Build history of the part. All positions in model axes, mm. Face numbers are marked on the shaded views. A direction names the side the tool comes from. Round coordinates to 2 decimals unless told otherwise and drop trailing zeros. Write each loop counter-clockwise with the first axis right and the second up, starting at its lowest first coordinate (ties: lowest second). Pieces come first, ordered by that corner, then holes.
Item 1: Band-saw the part on A-A, the plane x = 0. Write the cut outline in (y, z) (3 decimals).
Item 2: Band-saw the part on C-C, the plane y = 16. Write the cut outline in (x, z), then the cut area to 3 significant figures.
Item 3: 3-axis set-ups, long thin cutter, end or side, ignore diameter. For the marked faces 1, 2 and 3: which of +Z, -Z, +X, -X, +Y, -Y reach the whole face in a straight line?
Item 4: Mould opens along Z. For the marked faces 4, 5, 6 and 7 say: +Z half, -Z half, draft (parallel to the pull), parting line (faces both ways), or undercut.
Item 5: Band-saw the part on D-D, the plane y = 45. Write the cut outline in (x, z).
Item 6: Wall check: probe 1 along Z at (x, y) = (0, 3); probe 2 along X at (y, z) = (39, 0); probe 3 along Z at (x, y) = (0, 36). Give the ranges that are in metal, low to high.
Item 7: Drop flat-ended pins along their axis: pin 1 Ø13.5 at (x, z) = (-7.5, -4) entering from +Y; pin 2 Ø4 at (x, y) = (2, 38) entering from +Z; pin 3 Ø4 at (x, z) = (6.5, -31.5) entering from -Y; pin 4 Ø3 at (x, z) = (8, -36.5) entering from +Y. Give the stop position or say it passes through.
Item 8: Band-saw the part on B-B, the plane y = 34. Write the cut outline in (x, z), then the cut area to 3 significant figures.
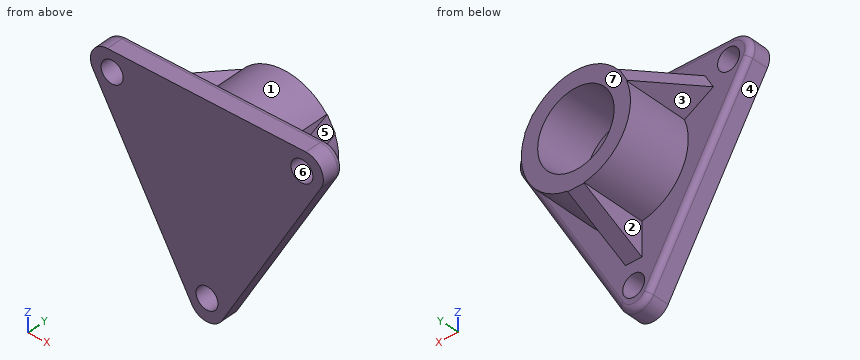
```python
from build123d import *

# Parameters (mm, degrees)
SKETCH1_R           = 6.369474113
SKETCH1_R_2         = 6.364401416
SKETCH1_R_3         = 6.413225573
BOSS_EXTRUDE2_DEPTH = 12.7
FILLET5_R           = 9.906
FILLET6_R           = 10.16
FILLET7_R           = 10.16
FILLET8_R           = 3.175
SKETCH2_R           = 31.696441514
BOSS_EXTRUDE3_DEPTH = 38.1
SKETCH3_R           = 22.193645705
CUT_EXTRUDE1_DEPTH  = 31.75
BOSS_EXTRUDE4_DEPTH = 4.7625
BOSS_EXTRUDE6_DEPTH = 9.525
CIRPATTERN1_COUNT   = 3


with BuildPart() as part:
    # Sketch1 → Boss-Extrude2 (new body)
    with BuildSketch(Plane(origin=(0, 0, 0), x_dir=(1, 0, 0), z_dir=(0, 1, 0))):
        Polygon((0, 86.591919686), (-74.990802211, -43.295959843), (74.990802211, -43.295959843), align=None)
        with Locations((0, 63.638807052)):
            Circle(SKETCH1_R, mode=Mode.SUBTRACT)
        with Locations((55.112823574, -31.819403526)):
            Circle(SKETCH1_R_2, mode=Mode.SUBTRACT)
        with Locations((-55.112823574, -31.819403526)):
            Circle(SKETCH1_R_3, mode=Mode.SUBTRACT)
    extrude(amount=BOSS_EXTRUDE2_DEPTH)

    # Fillet5
    fillet5_edges = [part.edges().sort_by_distance(p)[0] for p in [
        (-74.990802211, 6.35, 43.295959843),
    ]]
    fillet(fillet5_edges, radius=FILLET5_R)

    # Fillet6
    fillet6_edges = [part.edges().sort_by_distance(p)[0] for p in [
        (74.990802211, 6.35, 43.295959843),
    ]]
    fillet(fillet6_edges, radius=FILLET6_R)

    # Fillet7
    fillet7_edges = [part.edges().sort_by_distance(p)[0] for p in [
        (0, 6.35, -86.591919686),
    ]]
    fillet(fillet7_edges, radius=FILLET7_R)

    # Fillet8
    fillet8_edges = [part.edges().sort_by_distance(p)[0] for p in [
        (-0.219970453, 12.7, 43.295959843),
        (-66.411954561, 12.7, 38.342959843),
        (37.495401105, 12.7, -21.647979922),
        (66.191984109, 12.7, 38.215959843),
        (-37.605386332, 12.7, -21.457479922),
        (0, 12.7, -76.431919686),
    ]]
    fillet(fillet8_edges, radius=FILLET8_R)

    # Sketch2 → Boss-Extrude3 (add)
    with BuildSketch(Plane(origin=(0, 12.7, 0), x_dir=(1, 0, 0), z_dir=(0, 1, 0))):
        Circle(SKETCH2_R)
    extrude(amount=BOSS_EXTRUDE3_DEPTH)

    # Sketch3 → Cut-Extrude1 (cut)
    with BuildSketch(Plane(origin=(0, 50.8, 0), x_dir=(1, 0, 0), z_dir=(0, 1, 0))):
        Circle(SKETCH3_R)
    extrude(amount=-CUT_EXTRUDE1_DEPTH, mode=Mode.SUBTRACT)

    # Sketch6 → Boss-Extrude4 (add)
    with BuildSketch(Plane(origin=(0, 0, 0), x_dir=(-0.866025404, 0, 0.5), z_dir=(-0.5, 0, -0.866025404))):
        Polygon((31.696441514, 12.7), (50.655531139, 12.7), (31.696441514, 50.8), (28.066895326, 50.8), (28.066895326, 12.7), align=None)
    extrude(amount=BOSS_EXTRUDE4_DEPTH)

    # Sketch8 → Boss-Extrude6 (add)
    with BuildSketch(Plane(origin=(-2.38125, 0, -4.124445986), x_dir=(-0.866025404, 0, 0.5), z_dir=(-0.5, 0, -0.866025404))):
        Polygon((31.005254456, 12.578941577), (50.655531139, 12.7), (31.696441514, 50.8), (27.148658098, 50.8), (27.148658098, 12.578941577), align=None)
    boss_extrude6 = extrude(amount=-BOSS_EXTRUDE6_DEPTH)

    # CirPattern1: Boss-Extrude6 ×3 about axis
    cirpattern1_axis = Axis((0, 0, 0), (0, 1, 0))
    for i in range(1, CIRPATTERN1_COUNT):
        add(boss_extrude6.rotate(cirpattern1_axis, i * 360 / CIRPATTERN1_COUNT))


solid = part.part
```
Results:
1. outline: (0, -76.432) - (9.525, -76.432) arc R3.175 ccw to (12.7, -73.257) - (12.7, -70.008) - (0, -70.008) - close; (0, -57.269) - (12.7, -57.269) - (12.7, -50.656) - (50.8, -31.696) - (50.8, -22.194) - (19.05, -22.194) - (19.05, 22.194) - (50.8, 22.194) - (50.8, 31.696) - (12.7, 31.696) - (12.7, 40.121) arc R3.175 ccw to (9.525, 43.296) - (0, 43.296) - close
2. outline: (-44.83, 20.38) - (-29.52, 11.54) arc R31.7 ccw to (-4.76, -31.34) - (-4.76, -49.01) - (4.76, -49.01) - (4.76, -31.34) arc R31.7 ccw to (29.52, 11.54) - (44.83, 20.38) - (40.07, 28.63) - (24.76, 19.79) arc R31.7 ccw to (-24.76, 19.79) - (-40.07, 28.63) - close
2. area: 3,650 mm2
3. face 1: +Z, +Y
3. face 2: -Z, -X, +Y
3. face 3: -X, +Y
4. face 4: -Z half
4. face 5: +Z half
4. face 6: undercut
4. face 7: draft
5. outline: (-32.33, 13.17) - (-29.52, 11.54) arc R31.7 ccw to (-4.76, -31.34) - (-4.76, -34.58) - (4.76, -34.58) - (4.76, -31.34) arc R31.7 ccw to (29.52, 11.54) - (32.33, 13.17) - (27.57, 21.42) - (24.76, 19.79) arc R31.7 ccw to (-24.76, 19.79) - (-27.57, 21.42) - close; hole circle Ø44.39 at (0, 0)
6. probe 1: z = -76.43 to -70.01, -57.27 to 43.3
6. probe 2: x = -31.7 to -22.19, 22.19 to 31.7
6. probe 3: z = -39.06 to -22.19, 22.19 to 31.7
7. pin 1: stops at y = 19.05
7. pin 2: stops at z = 31.7
7. pin 3: stops at y = 0
7. pin 4: stops at y = 12.7
8. outline: (-37.07, 15.9) - (-29.52, 11.54) arc R31.7 ccw to (-4.76, -31.34) - (-4.76, -40.06) - (4.76, -40.06) - (4.76, -31.34) arc R31.7 ccw to (29.52, 11.54) - (37.07, 15.9) - (32.31, 24.15) - (24.76, 19.79) arc R31.7 ccw to (-24.76, 19.79) - (-32.31, 24.15) - close; hole circle Ø44.39 at (0, 0)
8. area: 1,850 mm2
